```python
from build123d import *

# Parameters (mm, degrees)
SKETCH1_R           = 2.1
BOSS_EXTRUDE2_DEPTH = 3
SKETCH1_14_R        = 5
CUT_EXTRUDE2_DEPTH  = 10
SKETCH2_R           = 4.5
CUT_EXTRUDE3_DEPTH  = 1.5


with BuildPart() as part:
    # Sketch1 → Boss-Extrude2 (new body)
    with BuildSketch(Plane(origin=(0, 0, 0), x_dir=(1, 0, 0), z_dir=(0, 1, 0))):
        with BuildLine():
            Line((32, -25), (32, -14.320549047))
            Line((32, -14.320549047), (28.692414075, -11.736497543))
            ThreePointArc((28.692414075, -11.736497543), (31, 0), (28.692414075, 11.736497543))
            Line((28.692414075, 11.736497543), (32, 14.320549047))
            Line((32, 14.320549047), (32, 25))
            Line((32, 25), (-32, 25))
            Line((-32, 25), (-32, 14.320549047))
            Line((-32, 14.320549047), (-28.692414075, 11.736497543))
            ThreePointArc((-28.692414075, 11.736497543), (-31, 0), (-28.692414075, -11.736497543))
            Line((-28.692414075, -11.736497543), (-32, -14.320549047))
            Line((-32, -14.320549047), (-32, -25))
            Line((-32, -25), (32, -25))
        make_face()
        with Locations(Location((26, 0, 0), (0, 0, 270))):
            Circle(SKETCH1_R, mode=Mode.SUBTRACT)
        with Locations(Location((-26, 0, 0), (0, 0, 270))):
            Circle(SKETCH1_R, mode=Mode.SUBTRACT)
    extrude(amount=BOSS_EXTRUDE2_DEPTH)

    # Sketch1_14 → Cut-Extrude2 (cut)
    with BuildSketch(Plane(origin=(0, 0, 0), x_dir=(1, 0, 0), z_dir=(0, 1, 0))):
        with Locations(Location((0, 0, 0), (0, 0, 270))):
            Circle(SKETCH1_14_R)
    extrude(amount=CUT_EXTRUDE2_DEPTH, mode=Mode.SUBTRACT)

    # Sketch2 → Cut-Extrude3 (cut)
    with BuildSketch(Plane(origin=(0, 3, 0), x_dir=(1, 0, 0), z_dir=(0, 1, 0))):
        with Locations(Location((4.75, 12, 0), (0, 0, 270))):
            Circle(SKETCH2_R)
        with Locations(Location((12.05, 17.5, 0), (0, 0, 270))):
            Circle(SKETCH2_R)
        with Locations(Location((4.75, -12, 0), (0, 0, 90))):
            Circle(SKETCH2_R)
        with Locations(Location((12.05, -17.5, 0), (0, 0, 90))):
            Circle(SKETCH2_R)
    extrude(amount=-CUT_EXTRUDE3_DEPTH, mode=Mode.SUBTRACT)


solid = part.part
```
The model under review builds one solid part; all positions refer to its coordinate system, in mm. A direction names the side the tool comes from. Round coordinates to 2 decimals unless told otherwise and drop trailing zeros. Write each loop counter-clockwise with the first axis right and the second up, starting at its lowest first coordinate (ties: lowest second). Pieces come first, ordered by that corner, then holes.
(1) Insertion check: pin 1 (7 mm diameter, centred on x = 12, z = 17.5, fed in from +Y); pin 2 (9 mm diameter, centred on x = 0, z = 0, fed in from +Y). Each pin has a flat end and moves straight along its axis. Give the tip position at first contact, or say it passes through.
(2) We need section D-D on z = -20. Give the boundary of the cut face in (x, y).
(3) Machinability: for faces 1 (the cylindrical face through (16.51, 2.26, -18.09)), 2 (the flat face through (0, 1, 25)), 3 (the flat face through (-30.32, 1.48, 13.01)), which of the approach directions +Z, -Z, +X, -X, +Y, -Y give a long, thin tool a straight path to every point of the face, cutting with its end or side? Answer none if there is none.
(4) We need section B-B on x = 1.5. Give the boundary of the cut face in (y, z), and give its area (3 significant figures).
(5) Wall thickness on L1, parallel to Z at x = 6, y = 2.45; L2, parallel to X at y = 2.1, z = 17.5; L3, parallel to Z at x = 0, y = 0.95: over which ranges is each line inside the solid? List them lowest first.
(6) We need section C-C on z = 18. Give the boundary of the cut face in (x, y), and give its area (3 significant figures).
(7) We need section A-A on y = 2.45. Give the boundary of the cut face in (x, z), and give its area (3 significant figures).
(8) Mouldability with a two-part tool opening along X and no side actions: class faces 4 (the flat face through (-30.369, 1.479, -13.047)), 5 (the flat face through (12, 1.5, -18)), 6 (the flat face through (-0.4, 3, 5.2)) as +X half, -X half, draft (parallel to the pull), parting line (faces both ways), or undercut.
Findings below:
1. pin 1: stops at y = 1.5
1. pin 2: passes through
2. outline: (-32, 0) - (32, 0) - (32, 3) - (15.79, 3) - (15.79, 1.5) - (8.31, 1.5) - (8.31, 3) - (-32, 3) - close
3. face 1: +Y
3. face 2: +Z, +X, -X, +Y, -Y
3. face 3: -X, +Y, -Y
4. outline: (0, -25) - (3, -25) - (3, -15.11) - (1.5, -15.11) - (1.5, -8.89) - (3, -8.89) - (3, -4.77) - (0, -4.77) - close; (0, 4.77) - (3, 4.77) - (3, 8.89) - (1.5, 8.89) - (1.5, 15.11) - (3, 15.11) - (3, 25) - (0, 25) - close
4. area: 103 mm2
5. L1: z = -25 to -16.32, -7.68 to 7.68, 16.32 to 25
5. L2: x = -32 to 7.55, 16.55 to 32
5. L3: z = -25 to -5, 5 to 25
6. outline: (-32, 0) - (32, 0) - (32, 3) - (16.52, 3) - (16.52, 1.5) - (7.58, 1.5) - (7.58, 3) - (-32, 3) - close
6. area: 179 mm2
7. outline: (-32, -25) - (32, -25) - (32, -14.32) - (28.69, -11.74) arc R31 ccw to (28.69, 11.74) - (32, 14.32) - (32, 25) - (-32, 25) - (-32, 14.32) - (-28.69, 11.74) arc R31 ccw to (-28.69, -11.74) - (-32, -14.32) - close; hole circle Ø4.2 at (-26, 0); hole circle Ø10 at (0, 0); hole circle Ø9 at (4.75, -12); hole circle Ø9 at (4.75, 12); hole circle Ø9 at (12.05, -17.5); hole circle Ø9 at (12.05, 17.5); hole circle Ø4.2 at (26, 0)
7. area: 2,740 mm2
8. face 4: -X half
8. face 5: undercut
8. face 6: draft
